Geometry: final body of the model. Coordinates: model frame, mm. Coordinates: 2 decimals unless noted, no trailing zeros. Loops run counter-clockwise (first coordinate to the right, second up) from the corner with the lowest first, then second, coordinate; pieces in that order, holes last. Notation, with made-up numbers: (80.25, 23.25) - (85.25, 23.25) arc R24 cw to (85.25, 55.25) - close; hole circle Ø4 at (13, 36.5). An arc over 180 degrees is marked (long way). Return JSON: item names as keys, results as strings.
from build123d import *

# Parameters (mm, degrees)
F2_DEPTH = 5
F3_R     = 10
F4_D     = 6


with BuildPart() as f2:
    # F1 (on Top) → F2 (new body)
    with BuildSketch(Plane.XY):
        Polygon((-25.0000044703, 65), (-65, -15), (-65, -65), (65, -65), (65, -15), (25, 65), align=None)
    extrude(amount=F2_DEPTH)

    # F3
    f3_edges = [f2.edges().sort_by_distance(p)[0] for p in [
        (-65, -65, 2.5),
        (-65, -15, 2.5),
        (-25.000004, 65, 2.5),
        (25, 65, 2.5),
        (65, -15, 2.5),
        (65, -65, 2.5),
    ]]
    fillet(f3_edges, radius=F3_R)

    # F4 (through all)
    with Locations(Plane(origin=(0, 0, 0), x_dir=(1, 0, 0), z_dir=(0, 0, -1))):
        with Locations((-55.0000044703, 25), (-25.0000044703, 25), (-55.0000044703, 55), (-25.0000044703, 55), (25, 55), (25, 25), (55, 25), (55, 55), (0, -50), (0, 55), (0, 25), (25, -15), (-2.2352e-06, -15), (-25.0000044703, -15)):
            Hole(F4_D / 2)


solid = f2.part
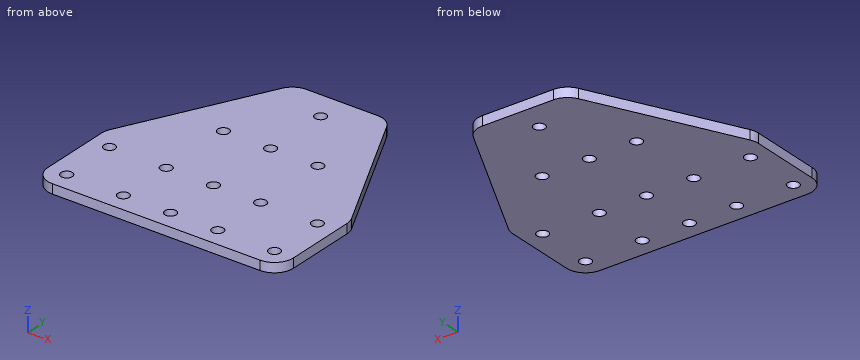
Item 1: Section query C-C, the plane y = -25. Return loops of the section in (x, z), and give its area (3 significant figures).
Worked out:
{"outline": "(-65, 0) - (-58, 0) - (-58, 5) - (-65, 5) - close; (-52, 0) - (-28, 0) - (-28, 5) - (-52, 5) - close; (-22, 0) - (-3, 0) - (-3, 5) - (-22, 5) - close; (3, 0) - (22, 0) - (22, 5) - (3, 5) - close; (28, 0) - (52, 0) - (52, 5) - (28, 5) - close; (58, 0) - (65, 0) - (65, 5) - (58, 5) - close", "area": "500 mm^2"}
Item 2: Section query D-D, the plane z = 3.9. Count the separate pieces of the cut face and the enclosed holes in it, and give its area (3 significant figures).
Worked out:
{"separate pieces": "1", "enclosed holes": "14", "area": "13,200 mm^2"}
Item 3: Section query B-B, the plane x = 0. Return loops of the section in (y, z), and give its area (3 significant figures).
Worked out:
{"outline": "(-65, 0) - (-58, 0) - (-58, 5) - (-65, 5) - close; (-52, 0) - (-28, 0) - (-28, 5) - (-52, 5) - close; (-22, 0) - (12, 0) - (12, 5) - (-22, 5) - close; (18, 0) - (47, 0) - (47, 5) - (18, 5) - close; (53, 0) - (65, 0) - (65, 5) - (53, 5) - close", "area": "530 mm^2"}
Item 4: First-contact query: pin 1 Ø5 at (x, y) = (0, -25) entering from +Z. Flat tip, straight axial feed; report the tip coordinate or a pass-through.
Worked out:
{"pin 1": "through"}
Item 5: Section query A-A, the plane y = 50. Return loops of the section in (x, z), and give its area (3 significant figures).
Worked out:
{"outline": "(-32.5, 0) - (-3, 0) - (-3, 5) - (-32.5, 5) - close; (3, 0) - (32.5, 0) - (32.5, 5) - (3, 5) - close", "area": "295 mm^2"}
Item 6: Ray query, probe 1 along Y at (x, z) = (0, 1.2); probe 2 along Y at (x, z) = (55, 3.85); probe 3 along X at (y, z) = (-55, 1.3). Return the intervals inside material, ascending. Write a range as from..to.
Worked out:
{"probe 1": "-65..-58, -52..-28, -22..12, 18..47, 53..65", "probe 2": "-65..-58, -52..-28, -22..5", "probe 3": "-65..-58, -52..-28, -22..-3, 3..22, 28..52, 58..65"}
